Can you work these out from the model? Positions are in its coordinate system, mm. Face numbers are marked on the shaded views. A direction names the side the tool comes from. Give positions to 0.01 mm unless a question says otherwise; leave off trailing zeros. Loops run counter-clockwise (first coordinate to the right, second up) from the corner with the lowest first, then second, coordinate; pieces in that order, holes last. Notation, with made-up numbers: M -37.75,87 L -4.75,87 A22 cw -4.75,112 Z; hole C 20,-14 d8. An arc over 180 degrees is marked long. Put each result on its own line as item: value. Start each with the question number.
1) If we mould it in two halves opening along Y, with no side actions, what happens to the marked faces 1, 2 and 3? For each: +Y half, -Y half, draft (parallel to the pull), parting line (faces both ways), or undercut.
2) Imagine slicing it at B-B (z = -1). State how many separate pieces and enclosed holes the cut face has, then the cut area to 3 significant figures.
3) Imagine slicing it at C-C (y = -3.5). Write out the boundary of the cut face in (x, z) (3 decimals).
4) Please list where these lines run through material, in increasing order: line 1 along Y through (x, z) = (-6.5, -2.8) (3 decimals); line 2 along X through (y, z) = (1.75, 0); line 3 along Z through (x, y) = (-4.25, 3.25). Write a range as from..to.
5) For the marked faces 4, 5 and 6, which set-ups out of +Z, -Z, +X, -X, +Y, -Y let a thin tool reach every point of the face, with its end or its side?
6) Imagine slicing it at A-A (y = 0). Write out the boundary of the cut face in (x, z) (3 decimals).
7) For P1, Ø1, axis at x = -8, z = 0, coming from the +Y side; P2, Ø1.6, axis at x = -6.5, y = 3.5, coming from the +Z side; P3, Ø2, axis at x = 6.5, z = 2, coming from the +Y side, each with a flat end and sliding along its axis, tell me the tip position at first contact or that it passes through.
8) Imagine slicing it at D-D (x = -6.25). Write out the boundary of the cut face in (y, z).
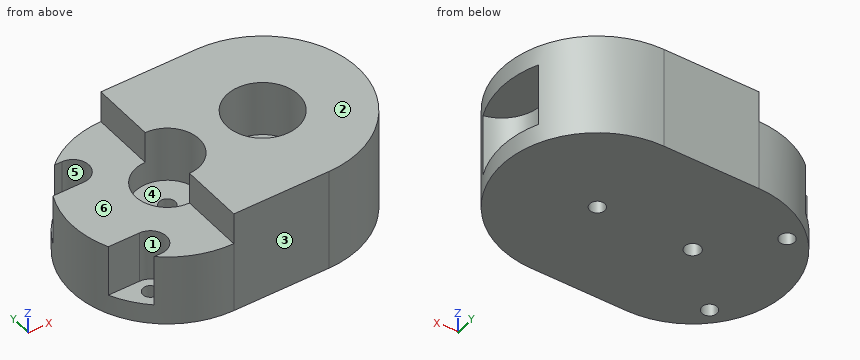
from build123d import *

# Parameters (mm, degrees)
SKETCH1_R                              = 0.5
BOSS_EXTRUDE1_DEPTH                    = 3.25
CUT_EXTRUDE1_DEPTH                     = 2
SKETCH3_W                              = 9.709711208
SKETCH3_H                              = 13.055758796
CUT_EXTRUDE2_DEPTH                     = 2
CUT_EXTRUDE3_DEPTH                     = 3.5
SKETCH5_R                              = 2.25
CUT_EXTRUDE4_DEPTH                     = 3.5
CUT_EXTRUDE5_DEPTH                     = 3.25
M1_2X0_25_TAPPED_HOLE1_D               = 0.95
M1_2X0_25_TAPPED_HOLE1_DEPTH           = 13.65
M1_2X0_25_TAPPED_HOLE1_TIP             = 0.285408794
M1_2X0_25_TAPPED_HOLE1_ON_FACE_2_D     = 0.95
M1_2X0_25_TAPPED_HOLE1_ON_FACE_2_DEPTH = 13.65
M1_2X0_25_TAPPED_HOLE1_ON_FACE_2_TIP   = 0.285408794


with BuildPart() as part:
    # Sketch1 → Boss-Extrude1 (new, symmetric)
    with BuildSketch(Plane.XY):
        with BuildLine():
            Line((-3, 6), (3, 6))
            ThreePointArc((3, 6), (9, 0), (3, -6))
            Line((3, -6), (-3, -6))
            ThreePointArc((-3, -6), (-9, 0), (-3, 6))
        make_face()
        with Locations((-3, 0)):
            Circle(SKETCH1_R, mode=Mode.SUBTRACT)
    extrude(amount=BOSS_EXTRUDE1_DEPTH, both=True)

    # Sketch2 → Cut-Extrude1 (cut, symmetric)
    with BuildSketch(Plane.XY):
        with BuildLine():
            ThreePointArc((8.454356057, 2.5), (6.454356057, 0), (8.454356057, -2.5))
            ThreePointArc((8.454356057, -2.5), (9, 0), (8.454356057, 2.5))
        make_face()
    extrude(amount=CUT_EXTRUDE1_DEPTH, both=True, mode=Mode.SUBTRACT)

    # Sketch3 → Cut-Extrude2 (cut)
    with BuildSketch(Plane.XY.offset(3.25)):
        with Locations((-7.854855604, -0.527879398)):
            Rectangle(SKETCH3_W, SKETCH3_H)
    extrude(amount=-CUT_EXTRUDE2_DEPTH, mode=Mode.SUBTRACT)

    # Sketch4 → Cut-Extrude3 (cut)
    with BuildSketch(Plane.XY.offset(3.25)):
        with BuildLine():
            ThreePointArc((-3, 2), (-5, 0), (-3, -2))
            ThreePointArc((-3, -2), (-1, 0), (-3, 2))
        make_face()
    extrude(amount=-CUT_EXTRUDE3_DEPTH, mode=Mode.SUBTRACT)

    # Sketch5 → Cut-Extrude4 (cut)
    with BuildSketch(Plane.XY.offset(3.25)):
        with Locations((3, 0)):
            Circle(SKETCH5_R)
    extrude(amount=-CUT_EXTRUDE4_DEPTH, mode=Mode.SUBTRACT)

    # Sketch6 → Cut-Extrude5 (cut)
    with BuildSketch(Plane.XY.offset(1.25)):
        with BuildLine():
            ThreePointArc((-6.5, -4.5), (-5.5, -3.5), (-6.5, -2.5))
            Line((-6.5, -2.5), (-8.454356057, -2.5))
            ThreePointArc((-8.454356057, -2.5), (-7.81644602, -3.577966983), (-6.968626967, -4.5))
            Line((-6.968626967, -4.5), (-6.5, -4.5))
        make_face()
        with BuildLine():
            ThreePointArc((-6.5, 2.5), (-5.5, 3.5), (-6.5, 4.5))
            Line((-6.5, 4.5), (-6.968626967, 4.5))
            ThreePointArc((-6.968626967, 4.5), (-7.81644602, 3.577966983), (-8.454356057, 2.5))
            Line((-8.454356057, 2.5), (-6.5, 2.5))
        make_face()
    extrude(amount=-CUT_EXTRUDE5_DEPTH, mode=Mode.SUBTRACT)

    # M1.2x0.25 Tapped Hole1
    with Locations(Plane(origin=(3, 0, -0.25), x_dir=(1, 0, 0), z_dir=(0, 0, 1))):
        with Locations((0, 0)):
            Hole(M1_2X0_25_TAPPED_HOLE1_D / 2, depth=M1_2X0_25_TAPPED_HOLE1_DEPTH)
            with Locations((0, 0, -(M1_2X0_25_TAPPED_HOLE1_DEPTH + M1_2X0_25_TAPPED_HOLE1_TIP / 2))):  # 118° drill point
                Cone(0, M1_2X0_25_TAPPED_HOLE1_D / 2, M1_2X0_25_TAPPED_HOLE1_TIP, mode=Mode.SUBTRACT)

    # M1.2x0.25 Tapped Hole1 on face 2
    with Locations(Plane(origin=(-6.5, 3.5, -2), x_dir=(1, 0, 0), z_dir=(0, 0, 1))):
        with Locations((0, 0), (0, -7)):
            Hole(M1_2X0_25_TAPPED_HOLE1_ON_FACE_2_D / 2, depth=M1_2X0_25_TAPPED_HOLE1_ON_FACE_2_DEPTH)
            with Locations((0, 0, -(M1_2X0_25_TAPPED_HOLE1_ON_FACE_2_DEPTH + M1_2X0_25_TAPPED_HOLE1_ON_FACE_2_TIP / 2))):  # 118° drill point
                Cone(0, M1_2X0_25_TAPPED_HOLE1_ON_FACE_2_D / 2, M1_2X0_25_TAPPED_HOLE1_ON_FACE_2_TIP, mode=Mode.SUBTRACT)


solid = part.part
Recorded:
1. face 1: undercut
1. face 2: draft
1. face 3: -Y half
2. separate pieces: 1
2. enclosed holes: 2
2. area: 166 mm²
3. outline: M -7.873,-3.25 L -6.975,-3.25 L -6.975,-2 L -7.873,-2 Z; M -6.025,-3.25 L 7.873,-3.25 L 7.873,3.25 L -3,3.25 L -3,1.25 L -5.5,1.25 L -5.5,-2 L -6.025,-2 Z
4. line 1: -4.873..-3.975, -3.025..3.025, 3.975..4.873
4. line 2: -8.74..-3.97, -2.03..1.59, 4.41..7.14
4. line 3: -3.25..1.25
5. face 4: +Z
5. face 5: +Z, -X
5. face 6: +Z, -X, +Y, -Y
6. outline: M -9,-3.25 L -3.5,-3.25 L -3.5,-0.25 L -5,-0.25 L -5,1.25 L -9,1.25 Z; M -2.5,-3.25 L 2.525,-3.25 L 2.525,-0.25 L 0.75,-0.25 L 0.75,3.25 L -1,3.25 L -1,-0.25 L -2.5,-0.25 Z; M 3.475,-3.25 L 9,-3.25 L 9,-2 L 6.454,-2 L 6.454,2 L 9,2 L 9,3.25 L 5.25,3.25 L 5.25,-0.25 L 3.475,-0.25 Z
7. P1: y = 2.5
7. P2: z = -2
7. P3: y = 5.45
8. outline: M -5.04,-3.25 L -3.9,-3.25 L -3.9,-2 L -4.47,-2 L -4.47,1.25 L -5.04,1.25 Z; M -3.1,-3.25 L 3.1,-3.25 L 3.1,-2 L 2.53,-2 L 2.53,1.25 L -2.53,1.25 L -2.53,-2 L -3.1,-2 Z; M 3.9,-3.25 L 5.04,-3.25 L 5.04,1.25 L 4.47,1.25 L 4.47,-2 L 3.9,-2 Z
